```python
from build123d import *

# Parameters (mm, degrees)
SALIENTE_EXTRUIR1_DEPTH = 3
CROQUIS2_R              = 2
CORTAR_EXTRUIR1_DEPTH   = 3


with BuildPart() as part:
    # Croquis1 → Saliente-Extruir1 (new body)
    with BuildSketch(Plane.XY):
        with BuildLine():
            ThreePointArc((16, 0), (9.177222982, -13.106432709), (-5.472322293, -15.035081933))
            Line((-5.472322293, -15.035081933), (-8.550503583, -23.49231552))
            ThreePointArc((-8.550503583, -23.49231552), (14.339410909, -20.478801107), (25, 0))
            ThreePointArc((25, 0), (14.339410909, 20.478801107), (-8.550503583, 23.49231552))
            Line((-8.550503583, 23.49231552), (-5.472322293, 15.035081933))
            ThreePointArc((-5.472322293, 15.035081933), (9.177222982, 13.106432709), (16, 0))
        make_face()
    extrude(amount=SALIENTE_EXTRUIR1_DEPTH)

    # Croquis2 → Cortar-Extruir1 (cut)
    with BuildSketch(Plane(origin=(0, 0, 0), x_dir=(-1, 0, 0), z_dir=(0, 0, -1))):
        with Locations((0, -19.5)):
            Circle(CROQUIS2_R)
        with Locations(Location((0, 19.5, 0), (0, 0, 180))):
            Circle(CROQUIS2_R)
    extrude(amount=-CORTAR_EXTRUIR1_DEPTH, mode=Mode.SUBTRACT)


solid = part.part
```
Input: part model. Units: mm. Frame: model coordinates. A direction names the side the tool comes from. Round coordinates to 2 decimals unless told otherwise and drop trailing zeros. Loops run counter-clockwise (first coordinate to the right, second up) from the corner with the lowest first, then second, coordinate; pieces in that order, holes last. Notation, with made-up numbers: (62, 42.5) - (92, 42.5) arc R9 cw to (92, 56.5) - close; hole circle Ø4 at (69.5, -27). An arc over 180 degrees is marked (long way). One line per item, written item: value. Start each with the question number.
(1) Ray query, line 1 (Y direction, x = 0, z = 2.2); line 2 (Y direction, x = -1.5, z = 2.2); line 3 (Y direction, x = 14, z = 1.15). Return the intervals inside material, ascending. Write a range as [from, to].
(2) Section C-C, the plane z = 0.9. Return loops of the section in (x, y).
(3) Section B-B, the plane y = 20. Return loops of the section in (x, z).
(4) Section D-D, the plane x = 15. Return loops of the section in (y, z), plus the area to 3 significant figures.
(5) Draft query along Y for faces 1 (the flat face through (15.4, -5.2, 3)), 2 (the cylindrical face through (-0.26, 17.517, 1.479)). Return one class per face: +Y half, -Y half, draft (parallel to the pull), parting line (faces both ways), or undercut.
(6) Contact query for flat-ended pins moving along their axis: P1, Ø5, axis at x = 2.5, y = 13.5, coming from the -Z side; P2, Ø1, axis at x = 11, y = 9.5, coming from the -Z side (3 decimals); P3, Ø1, axis at x = -3.5, z = 1, coming from the -Y side. Output: stop coordinate, or through.
(7) Section A-A, the plane x = 0. Return loops of the section in (y, z).
(8) Access query for faces 3 (the cylindrical face through (0.26, -17.517, 1.479)), 4 (the flat face through (-6.99, -19.2, 1.48)). Directions: +Z, -Z, +X, -X, +Y, -Y. A direction counts if a zero-diameter tool reaches every point of the face in a straight line with its end or side. Return the directions, or none.
Results below:
1. line 1: [-25, -21.5], [-17.5, -16], [16, 17.5], [21.5, 25]
1. line 2: [-24.95, -20.82], [-18.18, -15.93], [15.93, 18.18], [20.82, 24.95]
1. line 3: [-20.71, -7.75], [7.75, 20.71]
2. outline: (-8.55, -23.49) arc R25 ccw (long way) to (-8.55, 23.49) - (-5.47, 15.04) arc R16 cw (long way) to (-5.47, -15.04) - close; hole circle Ø4 at (0, -19.5); hole circle Ø4 at (0, 19.5)
3. outline: (-7.28, 0) - (-1.94, 0) - (-1.94, 3) - (-7.28, 3) - close; (1.94, 0) - (15, 0) - (15, 3) - (1.94, 3) - close
4. outline: (-20, 0) - (-5.57, 0) - (-5.57, 3) - (-20, 3) - close; (5.57, 0) - (20, 0) - (20, 3) - (5.57, 3) - close
4. area: 86.6 mm^2
5. face 1: draft
5. face 2: undercut
6. P1: z = 0
6. P2: through
6. P3: y = -24.82
7. outline: (-25, 0) - (-21.5, 0) - (-21.5, 3) - (-25, 3) - close; (-17.5, 0) - (-16, 0) - (-16, 3) - (-17.5, 3) - close; (16, 0) - (17.5, 0) - (17.5, 3) - (16, 3) - close; (21.5, 0) - (25, 0) - (25, 3) - (21.5, 3) - close
8. face 3: +Z, -Z
8. face 4: +Z, -Z, -X
